```python
from build123d import *

# Parameters (mm, degrees)
SKIZZE1_R                       = 80
AUFSATZ_LINEAR_AUSTRAGEN1_DEPTH = 15
SKIZZE8_R                       = 2.65
SCHNITT_LINEAR_AUSTRAGEN1_DEPTH = 15
KREISMUSTER1_COUNT              = 10
SKIZZE9_R                       = 4.5
SCHNITT_LINEAR_AUSTRAGEN2_DEPTH = 5
KREISMUSTER2_COUNT              = 10
AUFSATZ_LINEAR_AUSTRAGEN2_DEPTH = 15
KREISMUSTER3_COUNT              = 5
SKIZZE11_R                      = 2.6
SCHNITT_LINEAR_AUSTRAGEN3_DEPTH = 15


with BuildPart() as part:
    # Skizze1 → Aufsatz-Linear austragen1 (new body)
    with BuildSketch(Plane.XY):
        Circle(SKIZZE1_R)
    extrude(amount=AUFSATZ_LINEAR_AUSTRAGEN1_DEPTH)

    # Skizze8 → Schnitt-Linear austragen1 (cut)
    with BuildSketch(Plane(origin=(0, 0, 0), x_dir=(-1, 0, 0), z_dir=(0, 0, -1))):
        with Locations((0, -72.5)):
            Circle(SKIZZE8_R)
    schnitt_linear_austragen1 = extrude(amount=-SCHNITT_LINEAR_AUSTRAGEN1_DEPTH, mode=Mode.SUBTRACT)

    # Kreismuster1: Schnitt-Linear austragen1 ×10 about axis
    kreismuster1_axis = Axis((0, 0, 0), (0, 0, 1))
    for i in range(1, KREISMUSTER1_COUNT):
        add(schnitt_linear_austragen1.rotate(kreismuster1_axis, i * 360 / KREISMUSTER1_COUNT), mode=Mode.SUBTRACT)

    # Skizze9 → Schnitt-Linear austragen2 (cut)
    with BuildSketch(Plane(origin=(0, 0, 0), x_dir=(-1, 0, 0), z_dir=(0, 0, -1))):
        with Locations((0, -72.5)):
            Circle(SKIZZE9_R)
    schnitt_linear_austragen2 = extrude(amount=-SCHNITT_LINEAR_AUSTRAGEN2_DEPTH, mode=Mode.SUBTRACT)

    # Kreismuster2: Schnitt-Linear austragen2 ×10 about axis
    kreismuster2_axis = Axis((0, 0, 0), (0, 0, 1))
    for i in range(1, KREISMUSTER2_COUNT):
        add(schnitt_linear_austragen2.rotate(kreismuster2_axis, i * 360 / KREISMUSTER2_COUNT), mode=Mode.SUBTRACT)

    # Skizze10 → Aufsatz-Linear austragen2 (add)
    with BuildSketch(Plane.XY.offset(15)):
        with BuildLine():
            Line((-30, 69.852813742), (-30, 84.852813742))
            ThreePointArc((-30, 84.852813742), (0, 90), (30, 84.852813742))
            Line((30, 84.852813742), (30, 69.852813742))
            Line((30, 69.852813742), (0, 80))
            Line((0, 80), (-30, 69.852813742))
        make_face()
    aufsatz_linear_austragen2 = extrude(amount=-AUFSATZ_LINEAR_AUSTRAGEN2_DEPTH)

    # Kreismuster3: Aufsatz-Linear austragen2 ×5 about axis
    kreismuster3_axis = Axis((0, 0, 0), (0, 0, 1))
    for i in range(1, KREISMUSTER3_COUNT):
        add(aufsatz_linear_austragen2.rotate(kreismuster3_axis, i * 360 / KREISMUSTER3_COUNT))

    # Skizze11 → Schnitt-Linear austragen3 (cut)
    with BuildSketch(Plane.XY.offset(15)):
        with Locations((-15, 83.4)):
            Circle(SKIZZE11_R)
        with Locations((15, 83.4)):
            Circle(SKIZZE11_R)
    extrude(amount=-SCHNITT_LINEAR_AUSTRAGEN3_DEPTH, mode=Mode.SUBTRACT)


solid = part.part
```
Source: CAD feature listing. Evaluate the final solid. Frame: model axes, mm. A direction names the side the tool comes from. Give positions to 0.01 mm unless a question says otherwise; leave off trailing zeros. Loops run counter-clockwise (first coordinate to the right, second up) from the corner with the lowest first, then second, coordinate; pieces in that order, holes last. Notation, with made-up numbers: (2, 82.25) -> (52, 82.25) arc R11 ccw to (52, 103.25) -> close; hole circle Ø10 at (46, 12.25). An arc over 180 degrees is marked (long way). Put each result on its own line as item: value. Start each with the question number.
1) Cut plane A-A (x = 0). Return loops of the section in (y, z), then the cut area to 3 significant figures.
2) Draft query along X for faces 5 (the face through (-52.554, -73.062, 7.605)), 6 (the face through (53.246, -72.559, 7.605)), 7 (the face through (-22.42, -81.9, 7.6)), 8 (the face through (0, 90, 8)). Return one class per face: released by +X, released by -X, zero draft, split by the parting line, or undercut.
3) Cut plane D-D (x = 55). Return loops of the section in (y, z), then the cut area to 3 significant figures.
4) Cut plane B-B (y = -72.5). Return loops of the section in (x, z).
5) Reachability of faces 1 (the face through (-69.16, 25.045, 9.93)), 2 (the face through (66.274, 53.078, 7.605)), 3 (the face through (22.51, -82.02, 7.6)), 4 (the face through (-72.659, 19.854, 2.465)) from +Z, -Z, +X, -X, +Y, -Y: full face, straight path, thin tool, end or side. Return the list, or none.
6) Contact query for flat-ended pins moving along their axis: P1, Ø1, axis at y = -63, z = 4, coming from the -X side; P2, Ø7, axis at x = 68.95, y = 22.4, coming from the -Z side; P3, Ø3, axis at x = -27, z = 2, coming from the +Y side; P4, Ø7, axis at x = 42.61, y = 58.65, coming from the +Z side. Output: stop coordinate, or through.
7) Cut plane C-C (z = 10.5). State how many separate pieces and enclosed holes the cut face has, then the cut area to 3 significant figures.
8) Material intervals for probe 1 along X at (y, z) = (-23.5, 6.5); probe 2 along Y at (x, z) = (-71, 6.5); probe 3 along X at (y, z) = (82, 11.5), sorted ascending.
Results are:
1. outline: (-80, 0) -> (-77, 0) -> (-77, 5) -> (-75.15, 5) -> (-75.15, 15) -> (-80, 15) -> close; (-69.85, 5) -> (-68, 5) -> (-68, 0) -> (68, 0) -> (68, 5) -> (69.85, 5) -> (69.85, 15) -> (-69.85, 15) -> close; (75.15, 5) -> (77, 5) -> (77, 0) -> (90, 0) -> (90, 15) -> (75.15, 15) -> close
1. area: 2,350 mm2
2. face 5: released by -X
2. face 6: released by +X
2. face 7: undercut
2. face 8: split by the parting line
3. outline: (-71.24, 0) -> (58.09, 0) -> (58.09, 15) -> (-71.24, 15) -> close
3. area: 1,940 mm2
4. outline: (-53.33, 0) -> (-4.5, 0) -> (-4.5, 5) -> (-2.65, 5) -> (-2.65, 15) -> (-53.33, 15) -> close; (2.65, 5) -> (4.5, 5) -> (4.5, 0) -> (53.33, 0) -> (53.33, 15) -> (2.65, 15) -> close
5. face 1: +Z, -Z
5. face 2: +Z, -Z, +Y
5. face 3: +Z, -Z, -Y
5. face 4: -Z
6. P1: stops at x = -64.76
6. P2: stops at z = 5
6. P3: stops at y = 86.31
6. P4: stops at z = 15
7. separate pieces: 1
7. enclosed holes: 12
7. area: 22,900 mm2
8. probe 1: x = -76.47 to -71.36, -66.54 to 66.54, 71.36 to 76.47
8. probe 2: y = -55.31 to -46.68, -36.86 to -24.08, -20.72 to 20.72, 24.08 to 54.61
8. probe 3: x = -30 to -17.19, -12.81 to 12.81, 17.19 to 30
